from build123d import *

# Parameters (mm, degrees)
SKETCH2_R           = 12
CUT_EXTRUDE1_DEPTH  = 45
BOSS_EXTRUDE1_DEPTH = 10
SKETCH4_R           = 25
SKETCH4_R_2         = 15
BOSS_EXTRUDE2_DEPTH = 30


with BuildPart() as part:
    # Sketch1 → Revolve1 (revolve)
    with BuildSketch(Plane.XY):
        Polygon((0, 45), (0, 0), (37, 0), (25, 45), align=None)
    revolve(axis=Axis((0, 45, 0), (0, -1, 0)))

    # Sketch2 → Cut-Extrude1 (cut)
    with BuildSketch(Plane(origin=(0, 45, 0), x_dir=(1, 0, 0), z_dir=(0, 1, 0))):
        Circle(SKETCH2_R)
    extrude(amount=-CUT_EXTRUDE1_DEPTH, mode=Mode.SUBTRACT)

    # Sketch3 → Boss-Extrude1 (add, symmetric)
    with BuildSketch(Plane.XY):
        with BuildLine():
            Line((22, 0), (32, 0))
            Line((32, 0), (37.507136781, -20.552914271))
            ThreePointArc((37.507136781, -20.552914271), (39.650123165, -23.760120042), (43.302691739, -25))
            Line((43.302691739, -25), (50.574709256, -25))
            Line((50.574709256, -25), (50.574709256, -35))
            Line((50.574709256, -35), (32, -35))
            ThreePointArc((32, -35), (24.928932188, -32.071067812), (22, -25))
            Line((22, -25), (22, 0))
        make_face()
    extrude(amount=BOSS_EXTRUDE1_DEPTH, both=True)

    # Sketch4 → Boss-Extrude2 (add, symmetric)
    with BuildSketch(Plane.XY):
        with Locations((70, -35)):
            Circle(SKETCH4_R)
        with Locations((70, -35)):
            Circle(SKETCH4_R_2, mode=Mode.SUBTRACT)
    extrude(amount=BOSS_EXTRUDE2_DEPTH, both=True)


solid = part.part
The listing builds one solid part. Answer for the finished solid, in the listing's coordinates (mm). A direction names the side the tool comes from. Coordinates: 2 decimals unless noted, no trailing zeros. Write each loop counter-clockwise with the first axis right and the second up, starting at its lowest first coordinate (ties: lowest second). Pieces come first, ordered by that corner, then holes. Notation, with made-up numbers: M 43.25,-29.5 L 90.25,-29.5 A19 cw 90.25,-14.5 Z; hole C -38.75,-3 d3. An arc over 180 degrees is marked long. Put each result on its own line as item: value. Start each with the question number.
1. A cutting plane is placed at B-B on z = 0. Write down the section's boundary in (x, y), then the cut area to 3 significant figures.
2. For a pull along Y with two mould halves and no side action, classify faces 1 (the cylindrical face through (93.09, -44.58, 0.42)), 2 (the flat face through (32, -21, 10)), 3 (the cylindrical face through (58.944, -24.862, -0.42)), 4 (the flat face through (34.715, -10.133, 0.14)) as pulls with the +Y half, pulls with the -Y half, needs draft (parallel to the pull), parting line crosses it, or undercut.
3. Which of the six approach directions +Z, -Z, +X, -X, +Y, -Y give full straight-line access (tool end or side, diameter ignored) to faces 5 (the flat face through (45, -25, 0)), 6 (the flat face through (-6, 45, -11)), 7 (the flat face through (22, -13, 0))?
4. Flat-ended cylindrical pins translate along their axes: P1, Ø6.5, axis at x = 41, z = 3.5, coming from the -Y side; P2, Ø16, axis at y = -12, z = -1, coming from the -X side; P3, Ø1.1, axis at x = 45, z = 0, coming from the +Y side. Find the tip coordinate at first contact, or state that the pin passes through.
5. A cutting plane is placed at A-A on x = 70. Write down the section's boundary in (y, z), then the cut area to 3 significant figures.
6. A cutting plane is placed at D-D on y = -30. Write down the section's boundary in (x, z).
7. Consider line 1 (Y direction, x = 70, z = 0.5); line 2 (Y direction, x = -9.5, z = 11); line 3 (X direction, y = 22, z = 0). Determine where each line is inside the solid, lowest interval first. Write a range as from..to.
8. A cutting plane is placed at C-C on y = -46.5. Write down the section's boundary in (x, z).
Resolved:
1. outline: M -37,0 L -12,0 L -12,45 L -25,45 Z; M 12,0 L 22,0 L 22,-25 A10 ccw 32,-35 L 45,-35 A25 ccw long 47.09,-25 L 43.3,-25 A6 cw 37.51,-20.55 L 32,0 L 37,0 L 25,45 L 12,45 Z; hole C 70,-35 d30
1. area: 3,520 mm2
2. face 1: parting line crosses it
2. face 2: needs draft
2. face 3: undercut
2. face 4: undercut
3. face 5: +Z, -Z, +Y
3. face 6: +Z, -Z, +X, -X, +Y
3. face 7: +Z, -Z, -X, -Y
4. P1: stops at y = -35
4. P2: stops at x = 22
4. P3: stops at y = -25
5. outline: M -60,-30 L -50,-30 L -50,30 L -60,30 Z; M -20,-30 L -10,-30 L -10,30 L -20,30 Z
5. area: 1,200 mm2
6. outline: M 23.34,-10 L 45.51,-10 L 45.51,-30 L 55.86,-30 L 55.86,30 L 45.51,30 L 45.51,10 L 23.34,10 Z; M 84.14,-30 L 94.49,-30 L 94.49,30 L 84.14,30 Z
7. line 1: y = -60..-50, -20..-10
7. line 2: y = 0..45
7. line 3: x = -31.13..-12, 12..31.13
8. outline: M 47.8,-30 L 60.37,-30 L 60.37,30 L 47.8,30 Z; M 79.63,-30 L 92.2,-30 L 92.2,30 L 79.63,30 Z
